```python
from build123d import *

# Parameters (mm, degrees)
SKETCH_1_W          = 71.5
SKETCH_1_H          = 39
EXTRUDE_1_DEPTH     = 24.5
SKETCH_2_W          = 79.1
SKETCH_2_H          = 42.8
EXTRUDE_2_DEPTH     = 2
FILLET_1_R          = 0.7
FILLET_2_R          = 1
SKETCH_3_W          = 67.2
SKETCH_3_H          = 31.8
CUT_EXTRUDE_1_DEPTH = 1.2
SKETCH_4_R          = 6.4
EXTRUDE_3_DEPTH     = 12
SKETCH_5_W          = 28
SKETCH_5_H          = 28
CUT_EXTRUDE_2_DEPTH = 0.5


with BuildPart() as part:
    # Эскиз1 → Бобышка-Вытянуть1 (new body)
    with BuildSketch(Plane.XY):
        Rectangle(SKETCH_1_W, SKETCH_1_H)
    extrude(amount=EXTRUDE_1_DEPTH)

    # Эскиз2 → Бобышка-Вытянуть2 (add)
    with BuildSketch(Plane.XY.offset(24.5)):
        Rectangle(SKETCH_2_W, SKETCH_2_H)
    extrude(amount=EXTRUDE_2_DEPTH)

    # Скругление1
    fillet_1_edges = [part.edges().sort_by_distance(p)[0] for p in [
        (39.55, 0, 26.5),
        (0, 21.4, 26.5),
        (-39.55, 0, 26.5),
        (0, -21.4, 26.5),
    ]]
    fillet(fillet_1_edges, radius=FILLET_1_R)

    # Скругление2
    # the kernel refuses this fillet: 1 mm, written as the material it takes off along each edge
    with BuildSketch(Plane(origin=(-38.55, 20.4, 26.5), x_dir=(0, 1, 0), z_dir=(1, 0, 0))) as fillet_2_piece_1:
        with BuildLine():
            CenterArc((0.3, -0.7), 0.7, 0, 90)
            Line((1, -0.7), (1, 0))
            Line((1, 0), (0.3, 0))
        make_face()
    revolve(axis=Axis((-38.55, 20.4, 26.5), (0, 0, 1)), revolution_arc=90, mode=Mode.SUBTRACT)
    with BuildSketch(Plane(origin=(38.55, 20.4, 26.5), x_dir=(1, 0, 0), z_dir=(0, -1, 0))) as fillet_2_piece_2:
        with BuildLine():
            CenterArc((0.3, -0.7), 0.7, 0, 90)
            Line((1, -0.7), (1, 0))
            Line((1, 0), (0.3, 0))
        make_face()
    revolve(axis=Axis((38.55, 20.4, 26.5), (0, 0, 1)), revolution_arc=90, mode=Mode.SUBTRACT)
    with BuildSketch(Plane(origin=(-38.55, -20.4, 26.5), x_dir=(-1, 0, 0), z_dir=(0, 1, 0))) as fillet_2_piece_3:
        with BuildLine():
            CenterArc((0.3, -0.7), 0.7, 0, 90)
            Line((1, -0.7), (1, 0))
            Line((1, 0), (0.3, 0))
        make_face()
    revolve(axis=Axis((-38.55, -20.4, 26.5), (0, 0, 1)), revolution_arc=90, mode=Mode.SUBTRACT)
    with BuildSketch(Plane(origin=(38.55, -20.4, 26.5), x_dir=(0, -1, 0), z_dir=(-1, 0, 0))) as fillet_2_piece_4:
        with BuildLine():
            CenterArc((0.3, -0.7), 0.7, 0, 90)
            Line((1, -0.7), (1, 0))
            Line((1, 0), (0.3, 0))
        make_face()
    revolve(axis=Axis((38.55, -20.4, 26.5), (0, 0, 1)), revolution_arc=90, mode=Mode.SUBTRACT)
    with BuildSketch(Plane(origin=(39.55, -21.4, 22), x_dir=(0, 1, 0), z_dir=(0, 0, 1)), Plane(origin=(39.55, 21.4, 22), x_dir=(-1, 0, 0), z_dir=(0, 0, 1))) as fillet_2_piece_5:
        with BuildLine():
            CenterArc((FILLET_2_R, FILLET_2_R), FILLET_2_R, 180, 90)
            Line((0, FILLET_2_R), (0, 0))
            Line((0, 0), (FILLET_2_R, 0))
        make_face()
    extrude(amount=4.5, mode=Mode.SUBTRACT)
    with BuildSketch(Plane(origin=(-39.55, -21.4, 22), x_dir=(0, 1, 0), z_dir=(0, 0, 1)), Plane(origin=(-39.55, 21.4, 22), x_dir=(1, 0, 0), z_dir=(0, 0, 1))) as fillet_2_piece_6:
        with BuildLine():
            CenterArc((FILLET_2_R, -FILLET_2_R), FILLET_2_R, 90, 90)
            Line((0, -FILLET_2_R), (0, 0))
            Line((0, 0), (FILLET_2_R, 0))
        make_face()
    extrude(amount=4.5, mode=Mode.SUBTRACT)

    # Эскиз3 → Вырез-Вытянуть1 (cut)
    with BuildSketch(Plane.XY.offset(26.5)):
        Rectangle(SKETCH_3_W, SKETCH_3_H)
    extrude(amount=-CUT_EXTRUDE_1_DEPTH, mode=Mode.SUBTRACT)

    # Эскиз4 → Бобышка-Вытянуть3 (add)
    with BuildSketch(Plane.XY.offset(25.3)):
        with Locations((25.2, 5.4)):
            Circle(SKETCH_4_R)
    extrude(amount=EXTRUDE_3_DEPTH)

    # Эскиз5 → Вырез-Вытянуть2 (cut)
    with BuildSketch(Plane.XY.offset(25.3)):
        with Locations((-5.6, 0.282517759)):
            Rectangle(SKETCH_5_W, SKETCH_5_H)
    extrude(amount=-CUT_EXTRUDE_2_DEPTH, mode=Mode.SUBTRACT)


solid = part.part
```
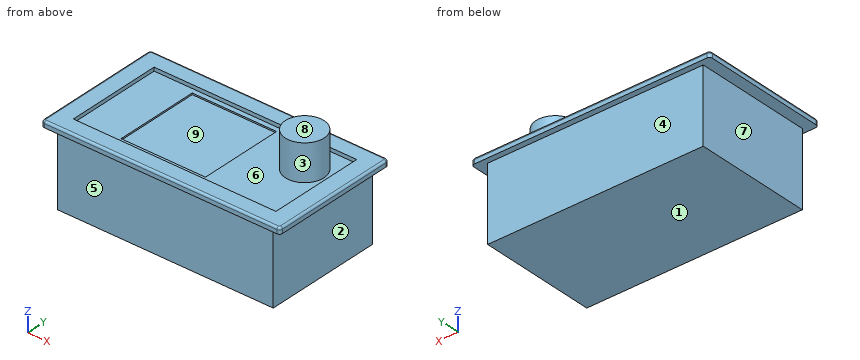
Part model, mm, in its own coordinate system. Face numbers are marked on the shaded views. A direction names the side the tool comes from. Round coordinates to 2 decimals unless told otherwise and drop trailing zeros. Loops run counter-clockwise (first coordinate to the right, second up) from the corner with the lowest first, then second, coordinate; pieces in that order, holes last.
1. 3-axis set-ups, long thin cutter, end or side, ignore diameter. For the marked faces 1, 2, 3, 4 and 5: which of +Z, -Z, +X, -X, +Y, -Y reach the whole face in a straight line?
Solutions:
face 1: -Z, +X, -X, +Y, -Y
face 2: -Z, +X, +Y, -Y
face 3: +Z
face 4: -Z, +X, -X, +Y
face 5: -Z, +X, -X, -Y
2. Slice it at B-B (x = -29.5). Give the cut face in (y, z), and give its area (3 significant figures).
Solutions:
outline: (-21.4, 24.5) - (-19.5, 24.5) - (-19.5, 0) - (19.5, 0) - (19.5, 24.5) - (21.4, 24.5) - (21.4, 25.8) arc R0.7 ccw to (20.7, 26.5) - (15.9, 26.5) - (15.9, 25.3) - (-15.9, 25.3) - (-15.9, 26.5) - (-20.7, 26.5) arc R0.7 ccw to (-21.4, 25.8) - close
area: 1,000 mm2
3. Drill centre lines: line 1 along Y through (x, z) = (21, 2); line 2 along X through (y, z) = (1.5, 3); line 3 along Z through (x, y) = (23, -2.5). Where is each one in solid material? Low to high.
Solutions:
line 1: y = -19.5 to 19.5
line 2: x = -35.75 to 35.75
line 3: z = 0 to 25.3
4. Slice it at C-C (z = 31.5). Give the cut face in (x, y), and give its area (3 significant figures).
Solutions:
outline: circle Ø12.8 at (25.2, 5.4)
area: 129 mm2
5. Flat gauge pins, fed straight in: pin 1 (1.5 mm diameter, centred on x = -27, y = -15, fed in from +Z); pin 2 (1 mm diameter, centred on x = 20, z = 15, fed in from +Y); pin 3 (6 mm diameter, centred on x = 31.5, y = -7, fed in from +Z). Where does each tip first touch, or does it go through?
Solutions:
pin 1: stops at z = 25.3
pin 2: stops at y = 19.5
pin 3: stops at z = 26.5
6. Slice it at A-A (y = 13). Give the cut face in (x, z).
Solutions:
outline: (-39.55, 24.5) - (-35.75, 24.5) - (-35.75, 0) - (35.75, 0) - (35.75, 24.5) - (39.55, 24.5) - (39.55, 25.8) arc R0.7 ccw to (38.85, 26.5) - (33.6, 26.5) - (33.6, 25.3) - (8.4, 25.3) - (8.4, 24.8) - (-19.6, 24.8) - (-19.6, 25.3) - (-33.6, 25.3) - (-33.6, 26.5) - (-38.85, 26.5) arc R0.7 ccw to (-39.55, 25.8) - close
7. Two-plate mould, pull along X, no slides. Class the marked faces 6, 7, 8 and 9: pulls with the +X half, pulls with the -X half, needs draft (parallel to the pull), parting line crosses it, or undercut.
Solutions:
face 6: undercut
face 7: pulls with the -X half
face 8: needs draft
face 9: undercut
8. Slice it at D-D (y = 5.4). Give the cut face in (x, z).
Solutions:
outline: (-39.55, 24.5) - (-35.75, 24.5) - (-35.75, 0) - (35.75, 0) - (35.75, 24.5) - (39.55, 24.5) - (39.55, 25.8) arc R0.7 ccw to (38.85, 26.5) - (33.6, 26.5) - (33.6, 25.3) - (31.6, 25.3) - (31.6, 37.3) - (18.8, 37.3) - (18.8, 25.3) - (8.4, 25.3) - (8.4, 24.8) - (-19.6, 24.8) - (-19.6, 25.3) - (-33.6, 25.3) - (-33.6, 26.5) - (-38.85, 26.5) arc R0.7 ccw to (-39.55, 25.8) - close
